from build123d import *

# Parameters (mm, degrees)
F0_W     = 99.410921
F0_H     = 55.796448
F1_DEPTH = 25.4
F2_W     = 50.8
F2_H     = 12.7
F3_DEPTH = 25.4
F4_W     = 19.05
F4_H     = 12.7
F5_DEPTH = 25.4
F7_R     = 6.35
F8_DEPTH = 101.6


with BuildPart() as f1:
    # F0 (on Front) → F1 (new body)
    with BuildSketch(Plane.XZ):
        with Locations((-49.705461, 27.898224)):
            Rectangle(F0_W, F0_H)
    extrude(amount=F1_DEPTH)

    # F2 (on face) → F3 (cut)
    with BuildSketch(Plane.XZ.offset(25.4)):
        with Locations((-50.8, 49.446448)):
            Rectangle(F2_W, F2_H)
    extrude(amount=-F3_DEPTH, mode=Mode.SUBTRACT)

    # F4 (on face) → F5 (cut)
    with BuildSketch(Plane.XZ.offset(25.4)):
        with Locations((-9.525, 6.35)):
            Rectangle(F4_W, F4_H)
    extrude(amount=-F5_DEPTH, mode=Mode.SUBTRACT)

    # F7 (on face) → F8 (cut)
    with BuildSketch(Plane.YZ):
        with Locations((-12.644938, 29.27478)):
            Circle(F7_R)
    extrude(amount=-F8_DEPTH, mode=Mode.SUBTRACT)


solid = f1.part
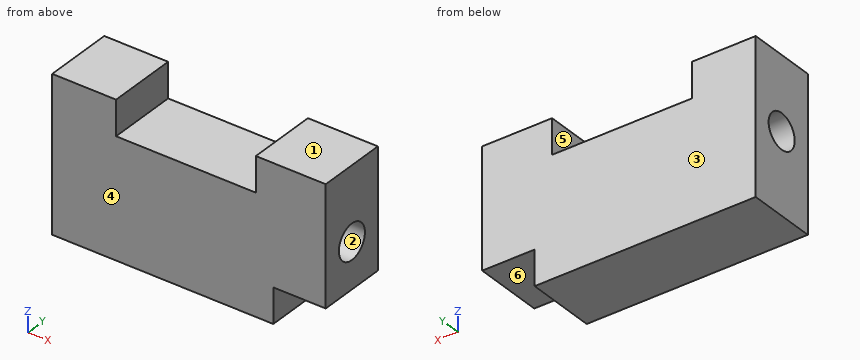
Work out the finished part from the listing and answer in its coordinate system (mm). Face numbers are marked on the shaded views. A direction names the side the tool comes from. Round coordinates to 2 decimals unless told otherwise and drop trailing zeros. Write each loop counter-clockwise with the first axis right and the second up, starting at its lowest first coordinate (ties: lowest second). Pieces come first, ordered by that corner, then holes.
1) A tool of negligible diameter and unlimited length cuts with its end or side. For the marked faces 4, 5 and 6, from which of +Z, -Z, +X, -X, +Y, -Y can it reach the whole face along a straight path? Write none if from no direction.
2) Given pin 1 Ø10 at (y, z) = (-17, 7.5) entering from +X; pin 2 Ø11.5 at (y, z) = (-12.64, 29.27) entering from +X, each flat-ended and moving along its own axis, determine where each tip first touches the part or whether it passes through.
3) A cutting plane is placed at C-C (x = -82.5). Give the vertices of the cut face in (y, z), plus the area to 3 significant figures.
4) The mould has two halves that part along Z. Classify the marked faces 1, 2 and 3: pulls with the +Z half, pulls with the -Z half, needs draft (parallel to the pull), parting line crosses it, or undercut.
5) A cutting plane is placed at B-B (z = 34.5). Give the vertices of the cut face in (x, y), plus the area to 3 significant figures.
6) Straight lines are drawn through the part: line 1 (Y direction, x = -49, z = 29.5); line 2 (X direction, y = -5, z = 47); line 3 (X direction, y = -13, z = 3). For each, find the intervals that lie inside material, in ascending order.
7) A cutting plane is placed at A-A (y = -11.75). Give the vertices of the cut face in (x, z).
8) A cutting plane is placed at D-D (y = -4). Give the vertices of the cut face in (x, z).
Completed:
1. face 4: +Z, -Z, +X, -X, -Y
1. face 5: +Z, +Y, -Y
1. face 6: -Z, +X, +Y, -Y
2. pin 1: stops at x = -19.05
2. pin 2: passes through
3. outline: (-25.4, 0) - (0, 0) - (0, 55.8) - (-25.4, 55.8) - close; hole circle Ø12.7 at (-12.64, 29.27)
3. area: 1,290 mm2
4. face 1: pulls with the +Z half
4. face 2: undercut
4. face 3: needs draft
5. outline: (-99.41, -25.4) - (0, -25.4) - (0, -16.25) - (-99.41, -16.25) - close; (-99.41, -9.04) - (0, -9.04) - (0, 0) - (-99.41, 0) - close
5. area: 1,810 mm2
6. line 1: y = -25.4 to -18.99, -6.3 to 0
6. line 2: x = -99.41 to -76.2, -25.4 to 0
6. line 3: x = -99.41 to -19.05
7. outline: (-99.41, 0) - (-19.05, 0) - (-19.05, 12.7) - (0, 12.7) - (0, 22.99) - (-99.41, 22.99) - close; (-99.41, 35.56) - (0, 35.56) - (0, 55.8) - (-25.4, 55.8) - (-25.4, 43.1) - (-76.2, 43.1) - (-76.2, 55.8) - (-99.41, 55.8) - close
8. outline: (-99.41, 0) - (-19.05, 0) - (-19.05, 12.7) - (0, 12.7) - (0, 55.8) - (-25.4, 55.8) - (-25.4, 43.1) - (-76.2, 43.1) - (-76.2, 55.8) - (-99.41, 55.8) - close
